from build123d import *

# Parameters (mm, degrees)
BOSS_EXTRUDE1_DEPTH = 20
SKETCH2_R           = 2.264817621
CUT_EXTRUDE1_DEPTH  = 3.25
SKETCH3_R           = 2.95
BOSS_EXTRUDE2_DEPTH = 5
SKETCH4_R           = 6.55
BOSS_EXTRUDE3_DEPTH = 1.5


with BuildPart() as part:
    # Sketch1 → Boss-Extrude1 (new body)
    with BuildSketch(Plane.XY):
        Polygon((0, 0), (40, 0), (40, 27.5), (47.325, 27.5), (47.325, 30.75), (40, 30.75), (40, 40.25), (0, 40.25), (0, 30.75), (-7.325, 30.75), (-7.325, 27.5), (0, 27.5), align=None)
    extrude(amount=BOSS_EXTRUDE1_DEPTH)

    # Sketch2 → Cut-Extrude1 (cut)
    with BuildSketch(Plane(origin=(0, 30.75, 0), x_dir=(1, 0, 0), z_dir=(0, 1, 0))):
        with Locations(Location((-4.3, -5.055444694, 0), (0, 0, 270))):
            Circle(SKETCH2_R)
        with Locations(Location((-4.3, -14.855444694, 0), (0, 0, 270))):
            Circle(SKETCH2_R)
        with Locations(Location((44.3, -14.855444694, 0), (0, 0, 270))):
            Circle(SKETCH2_R)
        with Locations(Location((44.3, -5.055444694, 0), (0, 0, 270))):
            Circle(SKETCH2_R)
    extrude(amount=-CUT_EXTRUDE1_DEPTH, mode=Mode.SUBTRACT)

    # Sketch3 → Boss-Extrude2 (add)
    with BuildSketch(Plane(origin=(0, 40.25, 0), x_dir=(1, 0, 0), z_dir=(0, 1, 0))):
        with Locations((30.15, -10)):
            Circle(SKETCH3_R)
    extrude(amount=BOSS_EXTRUDE2_DEPTH)

    # Sketch4 → Boss-Extrude3 (add)
    with BuildSketch(Plane(origin=(0, 40.25, 0), x_dir=(1, 0, 0), z_dir=(0, 1, 0))):
        with Locations((30.15, -10)):
            Circle(SKETCH4_R)
    extrude(amount=BOSS_EXTRUDE3_DEPTH)


solid = part.part
The model under review builds one solid part; all positions refer to its coordinate system, in mm. A direction names the side the tool comes from. Give positions to 0.01 mm unless a question says otherwise; leave off trailing zeros. Order: outer loops, then holes, each group sorted by start corner. A loop starts at its lowest first (then second) coordinate and runs counter-clockwise, first axis right, second up. Notation, with made-up numbers: M 63,-21 L 91,-21 A30 ccw 91,8 Z; hole C 3.5,44.25 d9. An arc over 180 degrees is marked long. Answer in a Markdown table with one row per item. Add a question column.
1. To check wall thickness, follow line 1 along Z through (x, y) = (-4, 28); line 2 along Y through (x, z) = (19.5, 19); line 3 along Y through (x, z) = (-2.5, 12.5). State the ranges of each line that lie inside material, in increasing order.
2. For pin 1 Ø10 at (y, z) = (9.5, 9.5) entering from +X; pin 2 Ø6 at (x, z) = (44, 6) entering from +Y; pin 3 Ø8 at (y, z) = (37, 14) entering from -X; pin 4 Ø12 at (x, y) = (14, 33.5) entering from -Z, all flat-tipped, find the tip position at first contact; note any pin that passes through.
3. Machinability: for faces 5 (the cylindrical face through (31.736, 43.476, 7.513)), 6 (the flat face through (0, 14, 10)), 7 (the flat face through (44, 30.75, 10)), 8 (the flat face through (-4, 30.75, 10)), 9 (the flat face through (30, 45.25, 10)), which of the approach directions +Z, -Z, +X, -X, +Y, -Y give a long, thin tool a straight path to every point of the face, cutting with its end or side? Answer none if there is none.
4. Mouldability with a two-part tool opening along Z and no side actions: class faces 1 (the cylindrical face through (46.546, 29.148, 4.761)), 2 (the flat face through (20, 20, 20)), 3 (the flat face through (-4, 27.5, 10)), 4 (the cylindrical face through (-5.68, 29.15, 13.06)) as released by +Z, released by -Z, zero draft, split by the parting line, or undercut.
5. Add section C-C on x = 30.15. State the section outline as (y, z) points.
6. Add section D-D on z = 10. State the section outline as (x, y) points (3 decimals), plus the area to 3 significant figures.
7. Add section A-A on x = -4.3. State the section outline as (y, z) points, plus the area to 3 significant figures.
8. Add section B-B on z = 15. State the section outline as (x, y) points (3 decimals), plus the area to 3 significant figures.
The answers:
| question | item | result |
|---|---|---|
| 1 | line 1 | 0 to 2.81, 7.3 to 12.61, 17.1 to 20 |
| 1 | line 2 | 0 to 40.25 |
| 1 | line 3 | 27.5 to 30.75 |
| 2 | pin 1 | x = 40 |
| 2 | pin 2 | y = 30.75 |
| 2 | pin 3 | x = 0 |
| 2 | pin 4 | z = 0 |
| 3 | face 5 | +Y |
| 3 | face 6 | +Z, -Z, -X, -Y |
| 3 | face 7 | +Z, -Z, +X, +Y |
| 3 | face 8 | +Z, -Z, -X, +Y |
| 3 | face 9 | +Z, -Z, +X, -X, +Y |
| 4 | face 1 | undercut |
| 4 | face 2 | released by +Z |
| 4 | face 3 | zero draft |
| 4 | face 4 | undercut |
| 5 | outline | M 0,0 L 40.25,0 L 40.25,3.45 L 41.75,3.45 L 41.75,7.05 L 45.25,7.05 L 45.25,12.95 L 41.75,12.95 L 41.75,16.55 L 40.25,16.55 L 40.25,20 L 0,20 Z |
| 6 | outline | M -7.325,27.5 L 0,27.5 L 0,0 L 40,0 L 40,27.5 L 47.325,27.5 L 47.325,30.75 L 40,30.75 L 40,40.25 L 36.7,40.25 L 36.7,41.75 L 33.1,41.75 L 33.1,45.25 L 27.2,45.25 L 27.2,41.75 L 23.6,41.75 L 23.6,40.25 L 0,40.25 L 0,30.75 L -7.325,30.75 Z |
| 6 | area | 1,700 mm2 |
| 7 | outline | M 27.5,0 L 30.75,0 L 30.75,2.79 L 27.5,2.79 Z; M 27.5,7.32 L 30.75,7.32 L 30.75,12.59 L 27.5,12.59 Z; M 27.5,17.12 L 30.75,17.12 L 30.75,20 L 27.5,20 Z |
| 7 | area | 35.6 mm2 |
| 8 | outline | M -7.325,27.5 L -6.56,27.5 L -6.56,30.75 L -7.325,30.75 Z; M -2.04,27.5 L 0,27.5 L 0,0 L 40,0 L 40,27.5 L 42.04,27.5 L 42.04,30.75 L 40,30.75 L 40,40.25 L 34.381,40.25 L 34.381,41.75 L 25.919,41.75 L 25.919,40.25 L 0,40.25 L 0,30.75 L -2.04,30.75 Z; M 46.56,27.5 L 47.325,27.5 L 47.325,30.75 L 46.56,30.75 Z |
| 8 | area | 1,640 mm2 |
